Answer from the drawing. Dimensions are ordinates in mm from the lowest x, y and z of the part. A direction names the side the tool comes from. Coordinates: 2 decimals unless noted, no trailing zeros. Order: outer loops, then holes, each group sorted by start corner. A loop starts at its lowest first (then second) coordinate and runs counter-clockwise, first axis right, second up. Notation, with made-up numbers: (-23, -13.75) - (10, -13.75) arc R10 ccw to (10, -3.75) - close; hole circle Ø8 at (74.5, -1.5). An arc over 180 degrees is marked (long way). One line per item, written item: value. Start each with the question number.
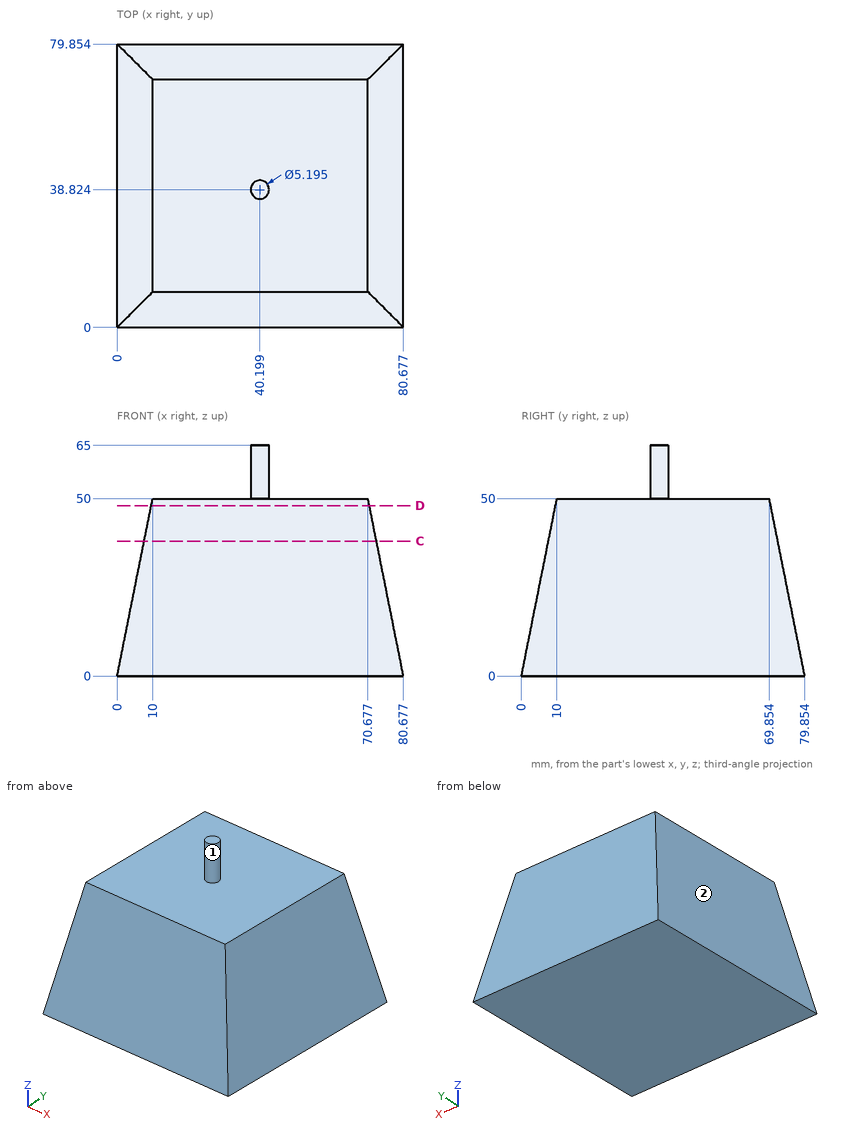
(1) Flat-ended cylindrical pins translate along their axes: pin 1 Ø1 at (x, y) = (20.5, 51) entering from +Z; pin 2 Ø18 at (x, y) = (29, 41.5) entering from +Z; pin 3 Ø4 at (x, z) = (59.5, 22.5) entering from -Y; pin 4 Ø12 at (x, z) = (42.5, 36.5) entering from +Y (1 decimal). Find the tip coordinate at first contact, or state that the pin passes through.
(2) Consider probe 1 along Z at (x, y) = (13, 23); probe 2 along X at (y, z) = (23, 39); probe 3 along X at (y, z) = (68.5, 23). Determine where each line is inside the solid, lowest interval first.
(3) For the marked faces 1 and 2, determine the directions among +Z, -Z, +X, -X, +Y, -Y from which every point of the face is accessible in a straight line to the end or side of a thin tool.
(4) The part is cut by section D-D on z = 48. Determine the outline of the cut face in (x, y) (1 decimal), plus the area to 3 significant figures.
(5) The part is cut by section C-C on z = 38. Determine the outline of the cut face in (x, y) (1 decimal), plus the area to 3 significant figures.
Completed:
1. pin 1: stops at z = 50
1. pin 2: stops at z = 65
1. pin 3: stops at y = 4.1
1. pin 4: stops at y = 73.8
2. probe 1: z = 0 to 50
2. probe 2: x = 7.8 to 72.88
2. probe 3: x = 4.6 to 76.08
3. face 1: +Z
3. face 2: +Z, -X, +Y, -Y
4. outline: (9.6, 9.6) - (71.1, 9.6) - (71.1, 70.3) - (9.6, 70.3) - close
4. area: 3,730 mm2
5. outline: (7.6, 7.6) - (73.1, 7.6) - (73.1, 72.3) - (7.6, 72.3) - close
5. area: 4,230 mm2
